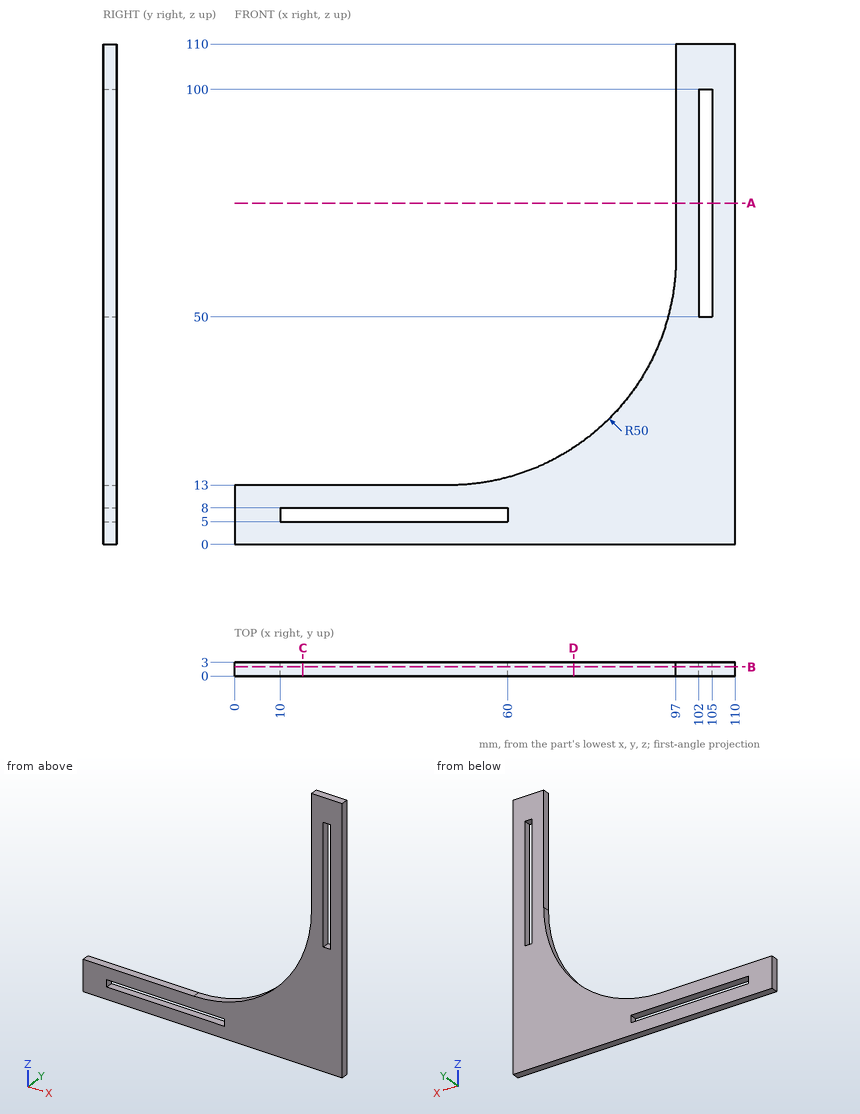
Study the drawing (mm; zero at the part's minimum x, y, z) and answer. Round coordinates to 2 decimals unless told otherwise and drop trailing zeros. Order: outer loops, then holes, each group sorted by start corner. A loop starts at its lowest first (then second) coordinate and runs counter-clockwise, first axis right, second up. Notation, with made-up numbers: (53.25, 44.25) - (91.25, 44.25) arc R10 cw to (91.25, 63.25) - close; hole circle Ø6 at (66, -38.5). An arc over 180 degrees is marked (long way). Use one line per item in the form item = value. Start each with the question number.
(1) Flat-ended cylindrical pins translate along their axes: pin 1 Ø1.5 at (x, y) = (48.5, 2) entering from -Z; pin 2 Ø1.5 at (y, z) = (1.5, 94.5) entering from -X; pin 3 Ø0.9 at (x, y) = (30.5, 1) entering from +Z. Find the tip coordinate at first contact, or state that the pin passes through.
(2) The part is cut by section A-A (z = 75). Give the vertices of the cut face in (x, y).
(3) The part is cut by section D-D (x = 74.5). Give the vertices of the cut face in (y, z).
(4) Find the intervals of material crossed by line 1 along Z through (x, y) = (104, 2.1); line 2 along Z through (x, y) = (16, 1.8); line 3 along X through (y, z) = (2.45, 73), in increasing order. Write a range as from..to.
(5) The part is cut by section C-C (x = 15). Give the vertices of the cut face in (y, z), then the cut area to 3 significant figures.
(6) The part is cut by section B-B (y = 2). Give the vertices of the cut face in (x, z).
Checked values:
q1.pin_1 = 0
q1.pin_2 = 97
q1.pin_3 = 13
q2.outline = (97, 0) - (102, 0) - (102, 3) - (97, 3) - close; (105, 0) - (110, 0) - (110, 3) - (105, 3) - close
q3.outline = (0, 0) - (3, 0) - (3, 21.24) - (0, 21.24) - close
q4.line_1 = 0..50, 100..110
q4.line_2 = 0..5, 8..13
q4.line_3 = 97..102, 105..110
q5.outline = (0, 0) - (3, 0) - (3, 5) - (0, 5) - close; (0, 8) - (3, 8) - (3, 13) - (0, 13) - close
q5.area = 30.0 mm^2
q6.outline = (0, 0) - (110, 0) - (110, 110) - (97, 110) - (97, 63) arc R50 cw to (47, 13) - (0, 13) - close; hole (10, 5) - (60, 5) - (60, 8) - (10, 8) - close; hole (102, 50) - (105, 50) - (105, 100) - (102, 100) - close
